from build123d import *

# Parameters (mm, degrees)
F1_DEPTH = 152.4
F2_W     = 140.266319
F2_H     = 52.757537
F3_DEPTH = 66.68789
F4_R     = 7.62
F5_DEPTH = 25.4
F4_R_2   = 12.3825
F6_DEPTH = 4.7625
F7_DEPTH = 25.4
F8_DEPTH = 2.2225
F9_DEPTH = 2.2225
F10_D    = 6.35
F11_R    = 1.27


with BuildPart() as f1:
    # F0 (on Right) → F1 (new body)
    with BuildSketch(Plane.YZ):
        Polygon((63.5, 0), (0, 0), (0, -76.2), (9.525, -76.2), (9.525, -66.280512), (63.5, -9.525), align=None)
    extrude(amount=F1_DEPTH)

    # F2 (on face) → F3 (cut)
    with BuildSketch(Plane(origin=(0, 0, -76.2), x_dir=(1, 0, 0), z_dir=(0, 0, -1))):
        with Locations((76.120947, -35.903768)):
            Rectangle(F2_W, F2_H)
    extrude(amount=-F3_DEPTH, mode=Mode.SUBTRACT)

    # F4 (on face) → F5 (cut)
    with BuildSketch(Plane.XY):
        with Locations((19.136649, 31.75)):
            Circle(F4_R)
    extrude(amount=-F5_DEPTH, mode=Mode.SUBTRACT)

    # F4 (on face) → F6 (cut)
    with BuildSketch(Plane.XY):
        with Locations((19.136649, 31.75)):
            Circle(F4_R_2)
        with Locations((19.136649, 31.75)):
            Circle(F4_R, mode=Mode.SUBTRACT)
    extrude(amount=-F6_DEPTH, mode=Mode.SUBTRACT)

    # F4 (on face) → F7 (cut)
    with BuildSketch(Plane.XY):
        with BuildLine():
            ThreePointArc((45.733401, 31.75), (55.258401, 22.225), (64.783401, 31.75))
            ThreePointArc((64.783401, 31.75), (55.258401, 41.275), (45.733401, 31.75))
        make_face()
    extrude(amount=-F7_DEPTH, mode=Mode.SUBTRACT)

    # F4 (on face) → F8 (cut)
    with BuildSketch(Plane.XY):
        with BuildLine():
            ThreePointArc((45.733401, 31.75), (55.258401, 41.275), (64.783401, 31.75))
            Line((64.783401, 31.75), (64.783401, 57.785))
            ThreePointArc((64.783401, 57.785), (64.039452, 59.581051), (62.243401, 60.325))
            Line((62.243401, 60.325), (48.273401, 60.325))
            ThreePointArc((48.273401, 60.325), (46.47735, 59.581051), (45.733401, 57.785))
            Line((45.733401, 57.785), (45.733401, 31.75))
        make_face()
    extrude(amount=-F8_DEPTH, mode=Mode.SUBTRACT)

    # F4 (on face) → F9 (cut)
    with BuildSketch(Plane.XY):
        with BuildLine():
            Line((64.783401, 5.715), (64.783401, 31.75))
            ThreePointArc((64.783401, 31.75), (55.258401, 22.225), (45.733401, 31.75))
            Line((45.733401, 31.75), (45.733401, 5.715))
            ThreePointArc((45.733401, 5.715), (46.47735, 3.918949), (48.273401, 3.175))
            Line((48.273401, 3.175), (62.243401, 3.175))
            ThreePointArc((62.243401, 3.175), (64.039452, 3.918949), (64.783401, 5.715))
        make_face()
    extrude(amount=-F9_DEPTH, mode=Mode.SUBTRACT)

    # F10 (through all)
    with Locations(Plane.XY):
        with Locations((82.797177, 50.8), (82.797177, 38.1), (82.797177, 25.4), (82.797177, 12.7)):
            Hole(F10_D / 2)

    # F11
    f11_edges = [f1.edges().sort_by_distance(p)[0] for p in [
        (152.4, 31.75, 0),
        (76.2, 63.5, 0),
        (0, 31.75, 0),
        (0, 63.5, -4.7625),
        (152.4, 63.5, -4.7625),
        (76.2, 63.5, -9.525),
    ]]
    fillet(f11_edges, radius=F11_R)


solid = f1.part
For this review, take the finished solid that the model builds, in its own axes (mm). A direction names the side the tool comes from. Give positions to 0.01 mm unless a question says otherwise; leave off trailing zeros. Loops run counter-clockwise (first coordinate to the right, second up) from the corner with the lowest first, then second, coordinate; pieces in that order, holes last. Notation, with made-up numbers: M -34,11.25 L 12,11.25 A9 cw 12,28.25 Z; hole C -14.75,50 d3. An arc over 180 degrees is marked long. Answer as a JSON object with one key per item and string values. Group by question number.
Q1. Add section B-B on y = 12.7. Give the boundary of the cut face in (x, z), and give its area (3 significant figures).
Q2. Mouldability with a two-part tool opening along X and no side actions: class faces 5 (the flat face through (152.4, 24, -30)), 6 (the flat face through (2.47, 36.21, -38.22)), 7 (the cylindrical face through (85.32, 36.17, -4.82)) as +X half, -X half, draft (parallel to the pull), parting line (faces both ways), or undercut.
Q3. Add section A-A on x = 84. Give the boundary of the cut face in (y, z) (3 decimals), and give its area (3 significant figures).
Q4. Add section D-D on z = -34. Give the boundary of the cut face in (x, y) (3 decimals), and give its area (3 significant figures).
Q5. Add section C-C on z = -56. Give the boundary of the cut face in (x, y) (3 decimals), and give its area (3 significant figures).
Q6. For probe 1 along X at (y, z) = (44, -17.5); probe 2 along X at (y, z) = (31, -3); probe 3 along Y at (x, z) = (132.5, -46) (3 decimals), list the stretches that pass through material, from the lowest coordinate up. Write a range as [from, to].
Q7. Tool access review of faces 1 (the flat face through (75, 36, -9.512)), 2 (the flat face through (149, 9.525, -71)), 3 (the flat face through (24.5, 37.4, -4.762)), 4 (the cylindrical face through (83.21, 53.95, -4.82)): name each direction out of +Z, -Z, +X, -X, +Y, -Y from which nothing blocks a thin tool from reaching the whole face with its end or side.
Q8. Insertion check: P1, Ø10, axis at x = 82.8, y = 50.8, coming from the -Z side; P2, Ø0.7, axis at x = 58.5, z = -1, coming from the +Y side; P3, Ø5.5, axis at x = 82.8, y = 12.7, coming from the +Z side; P4, Ø9.5, axis at x = 57, y = 42, coming from the +Z side. Each pin has a flat end and moves straight along its axis. Give the tip position at first contact, or say it passes through.
Checked values:
{
 "1": {"outline": "M 0,-62.94 L 5.99,-62.94 L 5.99,-9.51 L 79.62,-9.51 L 79.62,0 L 64.78,0 L 64.78,-2.22 L 45.73,-2.22 L 45.73,0 L 1.27,0 A1.27 ccw 0,-1.27 Z; M 85.97,-9.51 L 146.25,-9.51 L 146.25,-62.94 L 152.4,-62.94 L 152.4,-1.27 A1.27 ccw 151.13,0 L 85.97,0 Z", "area": "1,990 mm²"},
 "2": {"face 5": "+X half", "face 6": "draft", "face 7": "undercut"},
 "3": {"outline": "M 0,-76.2 L 9.525,-76.2 L 9.525,-9.512 L 9.762,-9.512 L 9.762,0 L 0,0 Z; M 15.638,-9.512 L 22.462,-9.512 L 22.462,0 L 15.638,0 Z; M 28.338,-9.512 L 35.162,-9.512 L 35.162,0 L 28.338,0 Z; M 41.038,-9.512 L 47.862,-9.512 L 47.862,0 L 41.038,0 Z; M 53.738,-9.512 L 62.283,-9.512 L 62.283,-10.805 L 63.15,-9.893 A1.27 ccw 63.5,-9.018 L 63.5,-1.27 A1.27 ccw 62.23,0 L 53.738,0 Z", "area": "1,020 mm²"},
 "4": {"outline": "M 0,0 L 152.4,0 L 152.4,40.224 L 146.254,40.224 L 146.254,9.525 L 5.988,9.525 L 5.988,40.224 L 0,40.224 Z", "area": "1,820 mm²"},
 "5": {"outline": "M 0,0 L 152.4,0 L 152.4,19.302 L 146.254,19.302 L 146.254,9.525 L 5.988,9.525 L 5.988,19.302 L 0,19.302 Z", "area": "1,570 mm²"},
 "6": {"probe 1": "[0, 5.99], [146.25, 152.4]", "probe 2": "[0, 6.78], [31.5, 45.76], [64.75, 152.4]", "probe 3": "[0, 9.525]"},
 "7": {"face 1": "-Z", "face 2": "-Z, +X, -X, +Y", "face 3": "+Z", "face 4": "+Z, -Z"},
 "8": {"P1": "z = -9.51", "P2": "y = 63.5", "P3": "through", "P4": "z = -2.22"}
}
